Could you check a few things on this drawing? It's one solid part, dimensions in mm from its lowest x, y, z. A direction names the side the tool comes from. Give positions to 0.01 mm unless a question says otherwise; leave off trailing zeros. Order: outer loops, then holes, each group sorted by start corner. A loop starts at its lowest first (then second) coordinate and runs counter-clockwise, first axis right, second up.
Item 1: Which directions (+Z, -Z, +X, -X, +Y, -Y) give clear straight access to the entire face, cutting with the end or side of a thin tool? Please do the marked faces 1 and 2.
Item 2: I want a section at A-A, the plane z = 5. Write out the boundary of the cut face in (x, y), then the cut area to 3 significant figures.
Item 3: I want a section at D-D, the plane z = 2.25. Write out the boundary of the cut face in (x, y), then the cut area to 3 significant figures.
Item 4: I want a section at B-B, the plane x = 3. Write out the boundary of the cut face in (y, z).
Item 5: I'm going to push flat-ended pins straight in: pin 1 Ø1 at (y, z) = (3, 3.5) entering from +X; pin 2 Ø1 at (x, y) = (5, 2) entering from -Z. Where does each tip first touch, or does it pass through?
Item 6: If I drill on line 1 along Y through (x, z) = (4.75, 9); line 2 along Z through (x, y) = (7, 2.25); line 3 along X through (y, z) = (2.7, 4.5), over which ranges is the centre line in solid material (lowest first)?
Item 7: I want a section at C-C, the plane y = 2. Write out the boundary of the cut face in (x, z), then the cut area to 3 significant figures.
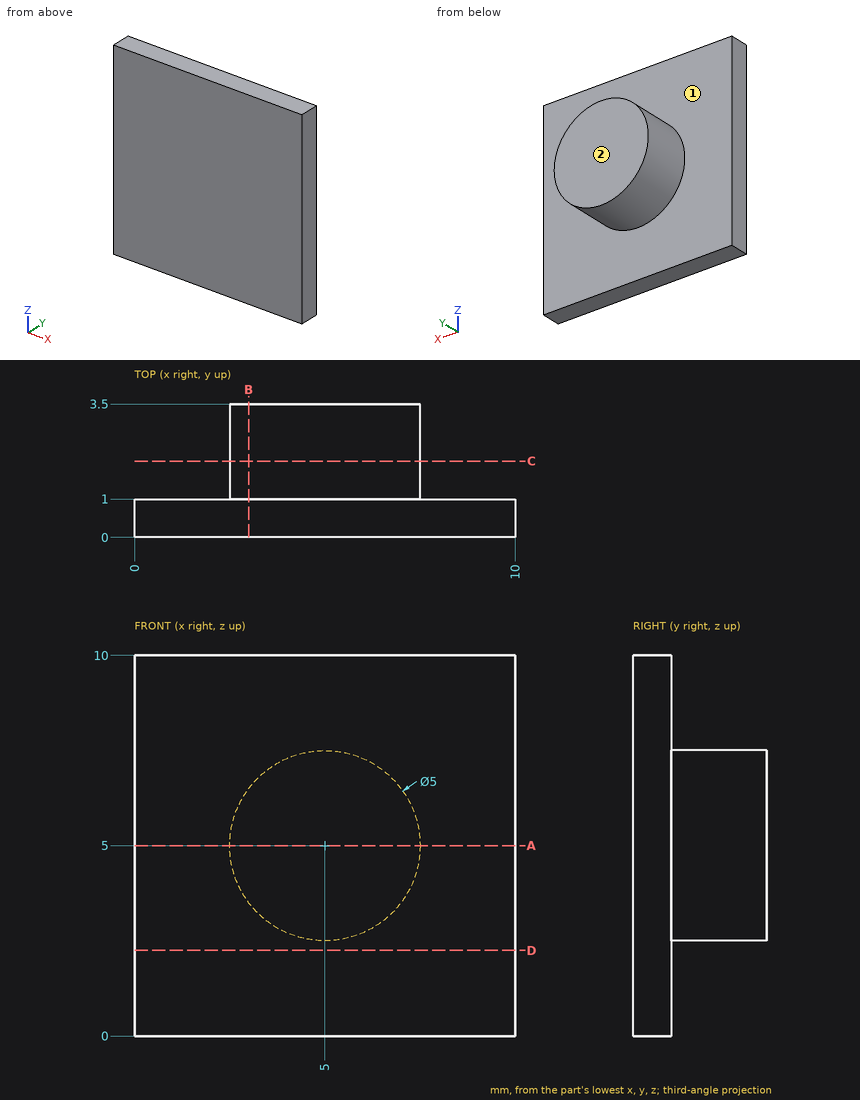
Results list:
1. face 1: +Y
1. face 2: +Z, -Z, +X, -X, +Y
2. outline: (0, 0) - (10, 0) - (10, 1) - (7.5, 1) - (7.5, 3.5) - (2.5, 3.5) - (2.5, 1) - (0, 1) - close
2. area: 22.5 mm2
3. outline: (0, 0) - (10, 0) - (10, 1) - (0, 1) - close
3. area: 10.0 mm2
4. outline: (0, 0) - (1, 0) - (1, 3.5) - (3.5, 3.5) - (3.5, 6.5) - (1, 6.5) - (1, 10) - (0, 10) - close
5. pin 1: stops at x = 7.29
5. pin 2: stops at z = 2.5
6. line 1: y = 0 to 1
6. line 2: z = 3.5 to 6.5
6. line 3: x = 2.55 to 7.45
7. outline: circle Ø5 at (5, 5)
7. area: 19.6 mm2
